from build123d import *

# Parameters (mm, degrees)
SKETCH_1_W              = 5
SKETCH_1_H              = 2.2
EXTRUDE_1_DEPTH         = 2.8
SKETCH_2_W              = 2.1
SKETCH_2_H              = 1.1
CUT_EXTRUDE_1_DEPTH     = 0.8
FILLET_1_R              = 0.5
MOVE_START              = -2.5
MOVE_BODY_1_DEPTH       = 5
MOVE_BODY_1_2_OUTLINE_W = 1.1
MOVE_BODY_1_2_OUTLINE_H = 0.8
MOVE_BODY_1_2_DEPTH     = 1.45
MOVE_START_2            = 1.05
MOVE_BODY_1_3_OUTLINE_W = 1.1
MOVE_BODY_1_3_OUTLINE_H = 0.8
MOVE_BODY_1_3_DEPTH     = 1.45
MOVE_BODY_1_4_DEPTH     = 5
MOVE_BODY_1_5_OUTLINE_W = 1.1
MOVE_BODY_1_5_OUTLINE_H = 0.8
MOVE_BODY_1_5_DEPTH     = 1.45
MOVE_BODY_1_6_OUTLINE_W = 1.1
MOVE_BODY_1_6_OUTLINE_H = 0.8
MOVE_BODY_1_6_DEPTH     = 1.45
SKETCH_3_W              = 1
SKETCH_3_H              = 1
EXTRUDE_2_DEPTH         = 1.8
SKETCH_4_W              = 1
SKETCH_4_H              = 1
EXTRUDE_3_DEPTH         = 1.8


# Read off the part's stored shape, not the designer's step: the move body step
with BuildPart() as part:
    # Sketch 1 → Extrude 1 (new body)
    with BuildSketch(Plane.XY):
        Rectangle(SKETCH_1_W, SKETCH_1_H)
    extrude(amount=EXTRUDE_1_DEPTH)

    # Sketch 2 → Cut-Extrude 1 (cut)
    with BuildSketch(Plane.XY.offset(2.8)):
        with Locations((0, -0.25)):
            Rectangle(SKETCH_2_W, SKETCH_2_H)
    extrude(amount=-CUT_EXTRUDE_1_DEPTH, mode=Mode.SUBTRACT)

    # Fillet 1
    fillet_1_edges = [part.edges().sort_by_distance(p)[0] for p in [
        (0, -1.1, 0),
        (0, 1.1, 0),
    ]]
    fillet(fillet_1_edges, radius=FILLET_1_R)



with BuildPart() as body_2:
    # Move Body 1 outline → Move Body 1 (new body)
    with BuildSketch(Plane.YZ.offset(MOVE_START)):
        with BuildLine():
            Line((9.1, 0.5), (9.1, 2.8))
            Line((9.1, 2.8), (8.3, 2.8))
            Line((8.3, 2.8), (8.3, 2))
            Line((8.3, 2), (7.2, 2))
            Line((7.2, 2), (7.2, 2.8))
            Line((7.2, 2.8), (6.9, 2.8))
            Line((6.9, 2.8), (6.9, 0.5))
            ThreePointArc((6.9, 0.5), (7.046446609, 0.146446609), (7.4, 0))
            Line((7.4, 0), (8.6, 0))
            ThreePointArc((8.6, 0), (8.953553391, 0.146446609), (9.1, 0.5))
        make_face()
    extrude(amount=MOVE_BODY_1_DEPTH)

    # Move Body 1 2 outline → Move Body 1 2 (add)
    with BuildSketch(Plane.YZ.offset(MOVE_START)):
        with Locations((7.75, 2.4)):
            Rectangle(MOVE_BODY_1_2_OUTLINE_W, MOVE_BODY_1_2_OUTLINE_H)
    extrude(amount=MOVE_BODY_1_2_DEPTH)

    # Move Body 1 3 outline → Move Body 1 3 (add)
    with BuildSketch(Plane.YZ.offset(MOVE_START_2)):
        with Locations((7.75, 2.4)):
            Rectangle(MOVE_BODY_1_3_OUTLINE_W, MOVE_BODY_1_3_OUTLINE_H)
    extrude(amount=MOVE_BODY_1_3_DEPTH)


with BuildPart() as body_3:
    # Move Body 1 4 outline → Move Body 1 4 (new body)
    with BuildSketch(Plane.YZ.offset(MOVE_START)):
        with BuildLine():
            Line((5.1, 0.5), (5.1, 2.8))
            Line((5.1, 2.8), (4.3, 2.8))
            Line((4.3, 2.8), (4.3, 2))
            Line((4.3, 2), (3.2, 2))
            Line((3.2, 2), (3.2, 2.8))
            Line((3.2, 2.8), (2.9, 2.8))
            Line((2.9, 2.8), (2.9, 0.5))
            ThreePointArc((2.9, 0.5), (3.046446609, 0.146446609), (3.4, 0))
            Line((3.4, 0), (4.6, 0))
            ThreePointArc((4.6, 0), (4.953553391, 0.146446609), (5.1, 0.5))
        make_face()
    extrude(amount=MOVE_BODY_1_4_DEPTH)

    # Move Body 1 5 outline → Move Body 1 5 (add)
    with BuildSketch(Plane.YZ.offset(MOVE_START)):
        with Locations((3.75, 2.4)):
            Rectangle(MOVE_BODY_1_5_OUTLINE_W, MOVE_BODY_1_5_OUTLINE_H)
    extrude(amount=MOVE_BODY_1_5_DEPTH)

    # Move Body 1 6 outline → Move Body 1 6 (add)
    with BuildSketch(Plane.YZ.offset(MOVE_START_2)):
        with Locations((3.75, 2.4)):
            Rectangle(MOVE_BODY_1_6_OUTLINE_W, MOVE_BODY_1_6_OUTLINE_H)
    extrude(amount=MOVE_BODY_1_6_DEPTH)


with BuildPart() as part_1:
    add(part.part)

    add(body_3.part)  # Extrude 2 merges body 3
    # Sketch 3 → Extrude 2 (add)
    with BuildSketch(Plane(origin=(0, 1.1, 0), x_dir=(1, 0, 0), z_dir=(0, 1, 0))):
        with Locations((-2, -2.3)):
            Rectangle(SKETCH_3_W, SKETCH_3_H)
        with Locations((2, -2.3)):
            Rectangle(SKETCH_3_W, SKETCH_3_H)
    extrude(amount=EXTRUDE_2_DEPTH)


    add(body_2.part)  # Extrude 3 merges body 2
    # Sketch 4 → Extrude 3 (add)
    with BuildSketch(Plane(origin=(0, 5.1, 0), x_dir=(1, 0, 0), z_dir=(0, 1, 0))):
        with Locations((2, -2.3)):
            Rectangle(SKETCH_4_W, SKETCH_4_H)
        with Locations((-2, -2.3)):
            Rectangle(SKETCH_4_W, SKETCH_4_H)
    extrude(amount=EXTRUDE_3_DEPTH)


solid = part_1.part
Could you check a few things on this model? Use its own coordinates, in mm. A direction names the side the tool comes from. Round coordinates to 2 decimals unless told otherwise and drop trailing zeros. Write each loop counter-clockwise with the first axis right and the second up, starting at its lowest first coordinate (ties: lowest second). Pieces come first, ordered by that corner, then holes. Notation, with made-up numbers: (-5, 74.5) -> (20, 74.5) arc R11 ccw to (20, 87.5) -> close; hole circle Ø4 at (-16.5, -12). An arc over 180 degrees is marked (long way). Use a Markdown table: item, result.
1. For pin 1 Ø0.5 at (x, y) = (2, 6) entering from -Z, with a flat end and sliding along its axis, tell me the tip position at first contact or that it passes through.
Answer key:
| item | result |
|---|---|
| pin 1 | stops at z = 1.8 |
2. Which directions (+Z, -Z, +X, -X, +Y, -Y) give clear straight access to the entire face, cutting with the end or side of a thin tool? Please do faces 1 (the face through (0, 0, 2)), 2 (the face through (-2, 6, 1.8)), 3 (the face through (1.5, 2, 2)).
Answer key:
| item | result |
|---|---|
| face 1 | +Z |
| face 2 | -Z, +X, -X |
| face 3 | +Z, -Z |
3. If we section it at B-B (z = 0.65): List the corners of the cut face in (x, y) for me.
Answer key:
| item | result |
|---|---|
| outline | (-2.5, -1.1) -> (2.5, -1.1) -> (2.5, 1.1) -> (-2.5, 1.1) -> close; (-2.5, 2.9) -> (2.5, 2.9) -> (2.5, 5.1) -> (-2.5, 5.1) -> close; (-2.5, 6.9) -> (2.5, 6.9) -> (2.5, 9.1) -> (-2.5, 9.1) -> close |
4. If we section it at D-D (y = 7.5): List the corners of the cut face in (x, z) for me.
Answer key:
| item | result |
|---|---|
| outline | (-2.5, 0) -> (2.5, 0) -> (2.5, 2.8) -> (1.05, 2.8) -> (1.05, 2) -> (-1.05, 2) -> (-1.05, 2.8) -> (-2.5, 2.8) -> close |
5. Please list where these lines run through material, in increasing order: probe 1 along Y at (x, z) = (1, 1.5); probe 2 along Y at (x, z) = (0.85, 2.2); probe 3 along X at (y, z) = (5.75, 2.1).
Answer key:
| item | result |
|---|---|
| probe 1 | y = -1.1 to 1.1, 2.9 to 5.1, 6.9 to 9.1 |
| probe 2 | y = -1.1 to -0.8, 0.3 to 1.1, 2.9 to 3.2, 4.3 to 5.1, 6.9 to 7.2, 8.3 to 9.1 |
| probe 3 | x = -2.5 to -1.5, 1.5 to 2.5 |
6. If we section it at C-C (y = 5.5): List the corners of the cut face in (x, z) for me.
Answer key:
| item | result |
|---|---|
| outline | (-2.5, 1.8) -> (-1.5, 1.8) -> (-1.5, 2.8) -> (-2.5, 2.8) -> close; (1.5, 1.8) -> (2.5, 1.8) -> (2.5, 2.8) -> (1.5, 2.8) -> close |
7. If we section it at A-A (x = -1.3): List the corners of the cut face in (y, z) for me.
Answer key:
| item | result |
|---|---|
| outline | (-1.1, 0.5) arc R0.5 ccw to (-0.6, 0) -> (0.6, 0) arc R0.5 ccw to (1.1, 0.5) -> (1.1, 2.8) -> (-1.1, 2.8) -> close; (2.9, 0.5) arc R0.5 ccw to (3.4, 0) -> (4.6, 0) arc R0.5 ccw to (5.1, 0.5) -> (5.1, 2.8) -> (2.9, 2.8) -> close; (6.9, 0.5) arc R0.5 ccw to (7.4, 0) -> (8.6, 0) arc R0.5 ccw to (9.1, 0.5) -> (9.1, 2.8) -> (6.9, 2.8) -> close |
8. We'd pull the mould along Y, two halves only. Please class faces 4 (the face through (0, 5.1, 1)), 5 (the face through (0, 8, 0)), 6 (the face through (2, 6, 1.8)): +Y half, -Y half, draft (parallel to the pull), parting line (faces both ways), or undercut.
Answer key:
| item | result |
|---|---|
| face 4 | undercut |
| face 5 | draft |
| face 6 | undercut |
